```python
from build123d import *

# Parameters (mm, degrees)
SKETCH1_R           = 12.288018633
SKETCH1_R_2         = 13.402342443
SKETCH1_R_3         = 5.966655134
BOSS_EXTRUDE1_DEPTH = 10


with BuildPart() as part:
    # Sketch1 → Boss-Extrude1 (new body)
    with BuildSketch(Plane.XY):
        with BuildLine():
            Line((-43.16670826, -100.459006624), (-43.16670826, -144.386357681))
            Line((-43.16670826, -144.386357681), (-43.16670826, -202.977586365))
            Line((-43.16670826, -202.977586365), (-19.89608029, -202.977586365))
            Line((-19.89608029, -202.977586365), (-19.89608029, -144.386357681))
            Line((-19.89608029, -144.386357681), (20.715262102, -144.386357681))
            Line((20.715262102, -144.386357681), (20.715262102, -202.977586365))
            Line((20.715262102, -202.977586365), (41.349988273, -202.977586365))
            Line((41.349988273, -202.977586365), (41.349988273, -144.386357681))
            Line((41.349988273, -144.386357681), (41.349988273, -100.459006624))
            Line((41.349988273, -100.459006624), (85.500022586, -100.459006624))
            Line((85.500022586, -100.459006624), (85.500022586, -144.386357681))
            Line((85.500022586, -144.386357681), (98.553668355, -144.386357681))
            Line((98.553668355, -144.386357681), (98.553668355, -100.459006624))
            Line((98.553668355, -100.459006624), (98.553668355, -85.011306082))
            Line((98.553668355, -85.011306082), (41.349988273, -85.011306082))
            Line((41.349988273, -85.011306082), (41.349988273, -57.873752711))
            ThreePointArc((41.349988273, -57.873752711), (1.129346742, 71.119036544), (-43.16670826, -56.531655566))
            Line((-43.16670826, -56.531655566), (-43.16670826, -85.011306082))
            Line((-43.16670826, -85.011306082), (-98.217954904, -85.011306082))
            Line((-98.217954904, -85.011306082), (-98.217954904, -100.459006624))
            Line((-98.217954904, -100.459006624), (-98.217954904, -143.510977861))
            Line((-98.217954904, -143.510977861), (-80.329625517, -143.510977861))
            Line((-80.329625517, -143.510977861), (-80.329625517, -100.459006624))
            Line((-80.329625517, -100.459006624), (-43.16670826, -100.459006624))
        make_face()
        with Locations((-33.517420804, 16.851364033)):
            Circle(SKETCH1_R, mode=Mode.SUBTRACT)
        with Locations((30.688490145, 16.851364033)):
            Circle(SKETCH1_R_2, mode=Mode.SUBTRACT)
        with Locations((0, -13.237752907)):
            Circle(SKETCH1_R_3, mode=Mode.SUBTRACT)
        with BuildLine():
            ThreePointArc((-47.4424626, -40.430436817), (0.125528844, -60.133744008), (47.693520288, -40.430436817))
            ThreePointArc((47.693520288, -40.430436817), (47.693520288, -27.743372786), (35.006456257, -27.743372786))
            ThreePointArc((35.006456257, -27.743372786), (0.125528844, -42.191525989), (-34.755398569, -27.743372786))
            ThreePointArc((-34.755398569, -27.743372786), (-47.4424626, -27.743372786), (-47.4424626, -40.430436817))
        make_face(mode=Mode.SUBTRACT)
    extrude(amount=BOSS_EXTRUDE1_DEPTH)


solid = part.part
```
For this review, take the finished solid that the model builds, in its own axes (mm). A direction names the side the tool comes from. Coordinates: 2 decimals unless noted, no trailing zeros. Write each loop counter-clockwise with the first axis right and the second up, starting at its lowest first coordinate (ties: lowest second). Pieces come first, ordered by that corner, then holes. Notation, with made-up numbers: (-36, 50) - (22, 50) arc R23 ccw to (22, 58) - close; hole circle Ø9 at (41, 73.25). An arc over 180 degrees is marked (long way). Put each result on its own line as item: value.
1. Add section A-A, the plane y = -173. Give the boundary of the cut face in (x, z), then the cut area to 3 significant figures.
Values found:
outline: (-43.17, 0) - (-19.9, 0) - (-19.9, 10) - (-43.17, 10) - close; (20.72, 0) - (41.35, 0) - (41.35, 10) - (20.72, 10) - close
area: 439 mm²
2. Add section C-C, the plane x = -54.5. Give the boundary of the cut face in (y, z).
Values found:
outline: (-100.46, 0) - (-85.01, 0) - (-85.01, 10) - (-100.46, 10) - close; (-45.7, 0) - (45.7, 0) - (45.7, 10) - (-45.7, 10) - close
3. For pin 1 (1 mm diameter, centred on x = -11.5, z = 1.5, fed in from +Y); pin 2 (4 mm diameter, centred on x = 20.5, z = 9, fed in from -Y); pin 3 (5 mm diameter, centred on x = 69, z = 4, fed in from -Y); pin 4 (3 mm diameter, centred on y = -78, z = 4.5, fed in from +X), all flat-tipped, find the tip position at first contact; note any pin that passes through.
Values found:
pin 1: y = 70.27
pin 2: y = -202.98
pin 3: y = -100.46
pin 4: x = 41.35
4. Machinability: for faces 4 (the flat face through (-89, -143.511, 5)), 5 (the flat face through (20.715, -173, 5)), 6 (the flat face through (41.35, -72, 5)), 7 (the cylindrical face through (0.67, -42.19, 4.93)), 8 (the flat face through (-43.167, -71, 5)), which of the approach directions +Z, -Z, +X, -X, +Y, -Y give a long, thin tool a straight path to every point of the face, cutting with its end or side? Answer none if there is none.
Values found:
face 4: +Z, -Z, -X, -Y
face 5: +Z, -Z, -Y
face 6: +Z, -Z, +X
face 7: +Z, -Z
face 8: +Z, -Z, -X
5. Wall thickness on probe 1 along Y at (x, z) = (0, 7); probe 2 along X at (y, z) = (-135.5, 4); probe 3 along X at (y, z) = (-185, 5.5): over which ranges is each line inside the solid? List them lowest first.
Values found:
probe 1: -144.39 to -60.13, -42.19 to -19.2, -7.27 to 71.13
probe 2: -98.22 to -80.33, -43.17 to 41.35, 85.5 to 98.55
probe 3: -43.17 to -19.9, 20.72 to 41.35
6. Mouldability with a two-part tool opening along X and no side actions: class faces 1 (the flat face through (31, -202.978, 5)), 2 (the flat face through (-98.218, -114, 5)), 3 (the cylindrical face through (-47.301, -27.605, 4.93)) as released by +X, released by -X, zero draft, split by the parting line, or undercut.
Values found:
face 1: zero draft
face 2: released by -X
face 3: undercut
7. Add section D-D, the plane z = 1.75. Give the boundary of the cut face in (x, y), then the cut area to 3 significant figures.
Values found:
outline: (-98.22, -143.51) - (-80.33, -143.51) - (-80.33, -100.46) - (-43.17, -100.46) - (-43.17, -202.98) - (-19.9, -202.98) - (-19.9, -144.39) - (20.72, -144.39) - (20.72, -202.98) - (41.35, -202.98) - (41.35, -100.46) - (85.5, -100.46) - (85.5, -144.39) - (98.55, -144.39) - (98.55, -85.01) - (41.35, -85.01) - (41.35, -57.87) arc R71.13 ccw (long way) to (-43.17, -56.53) - (-43.17, -85.01) - (-98.22, -85.01) - close; hole (-47.44, -40.43) arc R67.27 ccw to (47.69, -40.43) arc R8.97 ccw to (35.01, -27.74) arc R49.33 cw to (-34.76, -27.74) arc R8.97 ccw to start; hole circle Ø24.58 at (-33.52, 16.85); hole circle Ø11.93 at (0, -13.24); hole circle Ø26.8 at (30.69, 16.85)
area: 25,100 mm²
8. Add section B-B, the plane x = 0. Give the boundary of the cut face in (y, z), then the cut area to 3 significant figures.
Values found:
outline: (-144.39, 0) - (-60.13, 0) - (-60.13, 10) - (-144.39, 10) - close; (-42.19, 0) - (-19.2, 0) - (-19.2, 10) - (-42.19, 10) - close; (-7.27, 0) - (71.13, 0) - (71.13, 10) - (-7.27, 10) - close
area: 1,860 mm²
